```python
from build123d import *

# Parameters (mm, degrees)
SKETCH1_R           = 4
BOSS_EXTRUDE1_DEPTH = 10
CHAMFER1_SIZE       = 5


with BuildPart() as part:
    # Sketch1 → Boss-Extrude1 (new body)
    with BuildSketch(Plane.XY):
        Polygon((0, 150), (56.4, 150), (56.4, 100), (46.4, 100), (46.4, 50), (56.4, 50), (56.4, 0), (46.4, 0), (46.4, -137.127452116), (56.4, -137.127452116), (56.4, -332.021266673), (46.4, -332.021266673), (46.4, -365), (10, -365), (10, -332.021266673), (0, -332.021266673), (0, -137.127452116), (10, -137.127452116), (10, 0), (0, 0), (0, 50), (10, 50), (10, 100), (0, 100), align=None)
        with Locations((28.2, 75)):
            Circle(SKETCH1_R, mode=Mode.SUBTRACT)
        with Locations((28.2, -303.821266673)):
            Circle(SKETCH1_R, mode=Mode.SUBTRACT)
    extrude(amount=BOSS_EXTRUDE1_DEPTH)

    # Chamfer1
    chamfer1_edges = [part.edges().sort_by_distance(p)[0] for p in [
        (24.2, 75, 0),
        (24.2, -303.821266673, 0),
    ]]
    chamfer(chamfer1_edges, length=CHAMFER1_SIZE)


solid = part.part
```
Verification items for the finished model (mm, model axes). A direction names the side the tool comes from. Give positions to 0.01 mm unless a question says otherwise; leave off trailing zeros. Put each result on its own line as item: value.
Q1. Set-up check for faces 4 (the face through (10, -70, 5)), 5 (the face through (46.4, 75, 5)), 6 (the face through (46.4, -348, 5)): record each of +Z, -Z, +X, -X, +Y, -Y from which the full face is reachable in a straight line by a thin tool's end or side.
Result:
face 4: +Z, -Z, -X
face 5: +Z, -Z, +X
face 6: +Z, -Z, +X, -Y
Q2. Depth check by flat-ended pin: P1, Ø3, axis at y = -346.5, z = 4, coming from the +X side; P2, Ø4, axis at y = -42.5, z = 7.5, coming from the -X side; P3, Ø10, axis at x = 37.5, y = -257.5, coming from the -Z side; P4, Ø7, axis at x = 28.2, y = 75, coming from the +Z side. Enter the tip coordinate at first touch or a pass-through.
Result:
P1: x = 46.4
P2: x = 10
P3: z = 0
P4: through
Q3. Scan lines: probe 1 along Y at (x, z) = (28.2, 7.75); probe 2 along Y at (x, z) = (49, 6); probe 3 along X at (y, z) = (84.5, 2.5). Record each from-to range of solid material in increasing order. Write a range as from..to.
Result:
probe 1: -365..-307.82, -299.82..71, 79..150
probe 2: -332.02..-137.13, 0..50, 100..150
probe 3: 10..46.4
Q4. Mould release check, pull along Y, two halves, no side actions. Record for faces 1 (the face through (51, -137.127, 5)), 2 (the face through (10, -349, 5)), 3 (the face through (5, -332.021, 5)): released by +Y, released by -Y, zero draft, split by the parting line, or undercut.
Result:
face 1: undercut
face 2: zero draft
face 3: released by -Y
